```python
from build123d import *

# Parameters (mm, degrees)
SKETCH1_W            = 375
SKETCH1_H            = 420
BOSS_EXTRUDE1_DEPTH  = 6.35
FILLET1_R            = 10
M8_CLEARANCE_HOLE1_D = 9


with BuildPart() as part:
    # Sketch1 → Boss-Extrude1 (new body)
    with BuildSketch(Plane(origin=(0, 0, 0), x_dir=(1, 0, 0), z_dir=(0, 1, 0))):
        Rectangle(SKETCH1_W, SKETCH1_H)
    extrude(amount=BOSS_EXTRUDE1_DEPTH)

    # Fillet1
    fillet1_edges = [part.edges().sort_by_distance(p)[0] for p in [
        (187.5, 3.175, 210),
        (-187.5, 3.175, 210),
        (-187.5, 3.175, -210),
        (187.5, 3.175, -210),
    ]]
    fillet(fillet1_edges, radius=FILLET1_R)

    # M8 Clearance Hole1 (through all)
    with Locations(Plane(origin=(0, 6.35, 0), x_dir=(1, 0, 0), z_dir=(0, 1, 0))):
        with Locations((-77.5, -195), (62.5, -125), (-77.5, -125), (62.5, -195)):
            m8_clearance_hole1 = Hole(M8_CLEARANCE_HOLE1_D / 2)

    # Mirror1: M8 Clearance Hole1 across plane
    add(m8_clearance_hole1.mirror(Plane.XY), mode=Mode.SUBTRACT)


solid = part.part
```
Geometry: final body of the model. Coordinates: model frame, mm. Round coordinates to 2 decimals unless told otherwise and drop trailing zeros. Use CSV: the item, a comma, the result in double quotes. Start each with the question number.
1) Draft query along X for faces 1 (the face through (-3, 0, -3)), 2 (the face through (184.49, 3.22, 207.15)), 3 (the face through (-76.52, 3.13, 129.39)), 4 (the face through (-184.65, 3.22, 206.99)). Return one class per face: +X half, -X half, draft (parallel to the pull), parting line (faces both ways), or undercut.
2) Material intervals for line 1 along Z through (x, y) = (-77.5, 1.5); line 2 along X through (y, z) = (2, -125); line 3 along X through (y, z) = (3, 121.5), sorted ascending. Write a range as from..to.
3) First-contact query: pin 1 Ø8 at (x, z) = (-77.5, 195) entering from +Y. Flat tip, straight axial feed; report the tip coordinate or a pass-through.
Returned:
1,face 1,"draft"
1,face 2,"+X half"
1,face 3,"undercut"
1,face 4,"-X half"
2,line 1,"z = -210..-199.5, -190.5..-129.5, -120.5..120.5, 129.5..190.5, 199.5..210"
2,line 2,"x = -187.5..-82, -73..58, 67..187.5"
2,line 3,"x = -187.5..-80.33, -74.67..59.67, 65.33..187.5"
3,pin 1,"passes through"
